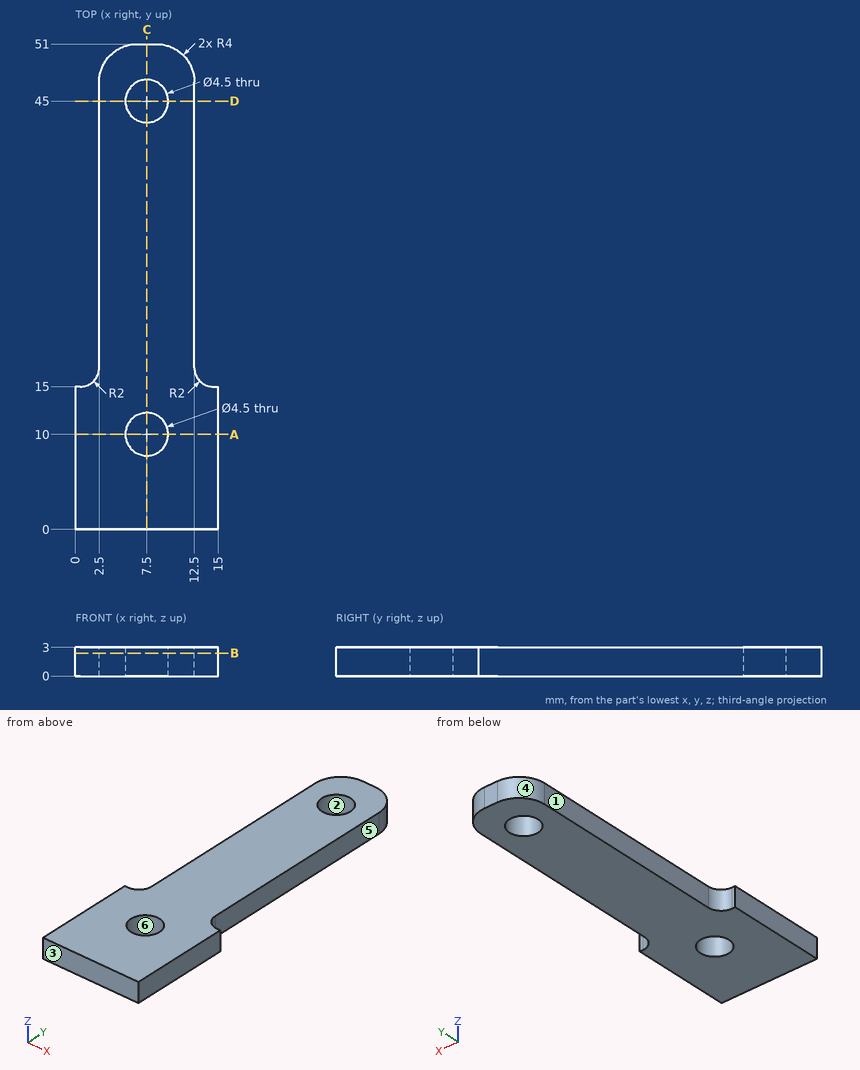
Geometry check sheet. Reference: drawing and pictorial views, mm from the part's lowest x, y, z. A direction names the side the tool comes from. Give positions to 0.01 mm unless a question says otherwise; leave off trailing zeros. Order: outer loops, then holes, each group sorted by start corner. A loop starts at its lowest first (then second) coordinate and runs counter-clockwise, first axis right, second up. Notation, with made-up numbers: M 38,40 L 45,40 A13 ccw 45,48 Z; hole C 79.5,5.25 d9. An arc over 180 degrees is marked long. Answer in a Markdown table with one row per item. Add a question column.
Q1. Sectioned sample at A-A, the plane y = 10. Record the boundary of the cut face in (x, z), and give its area (3 significant figures).
Q2. Gauge pin test, flat ends, axial feed: pin 1 Ø0.9 at (y, z) = (31, 1.5) entering from -X; pin 2 Ø1.5 at (x, z) = (10.5, 1.5) entering from +Y; pin 3 Ø1.5 at (y, z) = (25, 1) entering from +X. Record the tip position at first contact, or that the pin passes through.
Q3. Release check for a two-part mould opening along X. For the marked faces 3, 4, 5 and 6 record: released by +X, released by -X, zero draft, split by the parting line, or undercut.
Q4. Sectioned sample at B-B, the plane z = 2.4. Record the boundary of the cut face in (x, y).
Q5. Thickness scan on L1, parallel to Y at x = 7.5, z = 1.25; L2, parallel to Y at x = 6.25, z = 0.45; L3, parallel to X at y = 44, z = 1. Record the ranges inside material, lowest first.
Q6. Sectioned sample at C-C, the plane x = 7.5. Record the boundary of the cut face in (y, z).
Q7. Access from +Z, -Z, +X, -X, +Y, -Y to the whole of each face (thin tool, end or side, straight path). Record for the marked faces 1 and 2.
Q8. Sectioned sample at D-D, the plane y = 45. Record the boundary of the cut face in (x, z), and give its area (3 significant figures).
Verdict:
| question | item | result |
|---|---|---|
| 1 | outline | M 0,0 L 5.25,0 L 5.25,3 L 0,3 Z; M 9.75,0 L 15,0 L 15,3 L 9.75,3 Z |
| 1 | area | 31.5 mm² |
| 2 | pin 1 | x = 2.5 |
| 2 | pin 2 | y = 50.8 |
| 2 | pin 3 | x = 12.5 |
| 3 | face 3 | zero draft |
| 3 | face 4 | released by -X |
| 3 | face 5 | released by +X |
| 3 | face 6 | undercut |
| 4 | outline | M 0,0 L 15,0 L 15,15 L 14.5,15 A2 cw 12.5,17 L 12.5,47 A4 ccw 8.5,51 L 6.5,51 A4 ccw 2.5,47 L 2.5,17 A2 cw 0.5,15 L 0,15 Z; hole C 7.5,10 d4.5; hole C 7.5,45 d4.5 |
| 5 | L1 | 0 to 7.75, 12.25 to 42.75, 47.25 to 51 |
| 5 | L2 | 0 to 8.13, 11.87 to 43.13, 46.87 to 50.99 |
| 5 | L3 | 2.5 to 5.48, 9.52 to 12.5 |
| 6 | outline | M 0,0 L 7.75,0 L 7.75,3 L 0,3 Z; M 12.25,0 L 42.75,0 L 42.75,3 L 12.25,3 Z; M 47.25,0 L 51,0 L 51,3 L 47.25,3 Z |
| 7 | face 1 | +Z, -Z, -X, +Y |
| 7 | face 2 | +Z, -Z |
| 8 | outline | M 2.5,0 L 5.25,0 L 5.25,3 L 2.5,3 Z; M 9.75,0 L 12.5,0 L 12.5,3 L 9.75,3 Z |
| 8 | area | 16.5 mm² |
